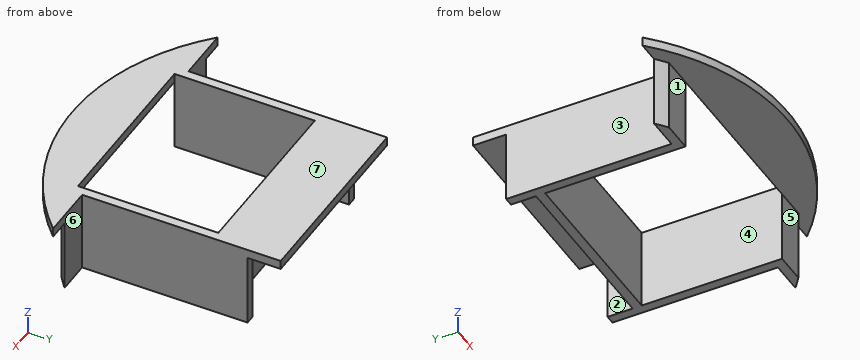
from build123d import *

# Parameters (mm, degrees)
BOSS_EXTRUDE2_DEPTH = 25.4
BOSS_EXTRUDE4_DEPTH = 25.4
SKETCH5_W           = 62.992
SKETCH5_H           = 49.022
BOSS_EXTRUDE5_DEPTH = 3.175


with BuildPart() as part:
    # Sketch2 → Boss-Extrude2 (new body)
    with BuildSketch(Plane.XY):
        Polygon((-34.671, -49.022), (-31.496, -49.022), (-31.496, 0), (31.496, 0), (31.496, -49.022), (34.671, -49.022), (34.671, 11.938), (31.496, 11.938), (31.496, 3.175), (-31.496, 3.175), (-31.496, 11.938), (-34.671, 11.938), align=None)
    extrude(amount=BOSS_EXTRUDE2_DEPTH)

    # Sketch4 → Boss-Extrude4 (add)
    with BuildSketch(Plane.XY.offset(25.4)):
        with BuildLine():
            Line((-34.671, -49.022), (-42.1386, -49.022))
            ThreePointArc((-42.1386, -49.022), (-44.170473584, -47.470511893), (-46.145273507, -45.847))
            Line((-46.145273507, -45.847), (-34.671, -45.847))
            Line((-34.671, -45.847), (-34.671, -49.022))
        make_face()
        with BuildLine():
            Line((34.671, -45.847), (34.671, -49.022))
            Line((34.671, -49.022), (42.1386, -49.022))
            ThreePointArc((42.1386, -49.022), (44.170473584, -47.470511893), (46.145273507, -45.847))
            Line((46.145273507, -45.847), (34.671, -45.847))
        make_face()
    extrude(amount=-BOSS_EXTRUDE4_DEPTH)

    # Sketch5 → Boss-Extrude5 (add)
    with BuildSketch(Plane.XY.offset(25.4)):
        with BuildLine():
            Line((-34.671, -45.847), (-34.671, 23.510170408))
            Line((-34.671, 23.510170408), (34.671, 23.510170408))
            Line((34.671, 23.510170408), (34.671, -45.847))
            Line((34.671, -45.847), (53.64486804, -45.847))
            ThreePointArc((53.64486804, -45.847), (0, -67.929829592), (-53.64486804, -45.847))
            Line((-53.64486804, -45.847), (-34.671, -45.847))
        make_face()
        with Locations((0, -24.511)):
            Rectangle(SKETCH5_W, SKETCH5_H, mode=Mode.SUBTRACT)
    extrude(amount=BOSS_EXTRUDE5_DEPTH)


solid = part.part
Check sheet for the modelled part. Datum: model origin and axes. Units: mm. Face numbers are marked on the shaded views. A direction names the side the tool comes from. Give positions to 0.01 mm unless a question says otherwise; leave off trailing zeros. Write each loop counter-clockwise with the first axis right and the second up, starting at its lowest first coordinate (ties: lowest second). Pieces come first, ordered by that corner, then holes. Notation, with made-up numbers: (58.25, 46.25) -> (77.25, 46.25) arc R21 ccw to (77.25, 79.25) -> close; hole circle Ø11 at (-29.5, -32.75). An arc over 180 degrees is marked (long way). Use one line per item in the form item = value. Start each with the question number.
1. Access from +Z, -Z, +X, -X, +Y, -Y to the whole of each face (thin tool, end or side, straight path). Record for the marked faces 5, 6 and 7.
2. Thickness scan on line 1 along X through (y, z) = (8.5, 3.25); line 2 along Y through (x, z) = (-30, 24.5) (3 decimals); line 3 along Y through (x, z) = (33.5, 21). Record the ranges inside material, lowest first. Write a range as from..to.
3. Section check B-B (x = -6). Record the cut outline in (y, z) (3 decimals), and give its area (3 significant figures).
4. Mould release check, pull along X, two halves, no side actions. Record for the marked faces 1, 2, 3 and 4: pulls with the +X half, pulls with the -X half, needs draft (parallel to the pull), parting line crosses it, or undercut.
5. Section check C-C (z = 5). Record the cut outline in (x, y) (3 decimals).
6. Go/stop test with flat-tipped pins: P1, Ø3, axis at x = -23, z = 14.5, coming from the -Y side; P2, Ø17.5, axis at x = -25.5, y = -57.5, coming from the -Z side; P3, Ø2, axis at x = -34, z = 15.5, coming from the -Y side. Record where each tip stops, or that it passes through.
7. Section check A-A (y = -3.5). Record the cut outline in (x, z) (3 decimals).
8. Section check D-D (y = 6.5). Record the cut outline in (x, z) (3 decimals), and give its area (3 significant figures).
Conclusion:
q1.face_5 = -Z, +X, -X, -Y
q1.face_6 = +Z, -Z, +X, +Y
q1.face_7 = +Z, +X, -X, +Y, -Y
q2.line_1 = -34.67..-31.5, 31.5..34.67
q2.line_2 = 0..3.175
q2.line_3 = -49.02..11.94
q3.outline = (-67.693, 25.4) -> (-49.022, 25.4) -> (-49.022, 28.575) -> (-67.693, 28.575) -> close; (0, 0) -> (3.175, 0) -> (3.175, 25.4) -> (23.51, 25.4) -> (23.51, 28.575) -> (0, 28.575) -> close
q3.area = 215 mm²
q4.face_1 = needs draft
q4.face_2 = undercut
q4.face_3 = pulls with the -X half
q4.face_4 = undercut
q5.outline = (-46.145, -45.847) arc R71.12 ccw to (-42.139, -49.022) -> (-31.496, -49.022) -> (-31.496, 0) -> (31.496, 0) -> (31.496, -49.022) -> (42.139, -49.022) arc R71.12 ccw to (46.145, -45.847) -> (34.671, -45.847) -> (34.671, 11.938) -> (31.496, 11.938) -> (31.496, 3.175) -> (-31.496, 3.175) -> (-31.496, 11.938) -> (-34.671, 11.938) -> (-34.671, -45.847) -> close
q6.P1 = 0
q6.P2 = 25.4
q6.P3 = -49.02
q7.outline = (-34.671, 0) -> (-31.496, 0) -> (-31.496, 28.575) -> (-34.671, 28.575) -> close; (31.496, 0) -> (34.671, 0) -> (34.671, 28.575) -> (31.496, 28.575) -> close
q8.outline = (-34.671, 0) -> (-31.496, 0) -> (-31.496, 25.4) -> (31.496, 25.4) -> (31.496, 0) -> (34.671, 0) -> (34.671, 28.575) -> (-34.671, 28.575) -> close
q8.area = 381 mm²
